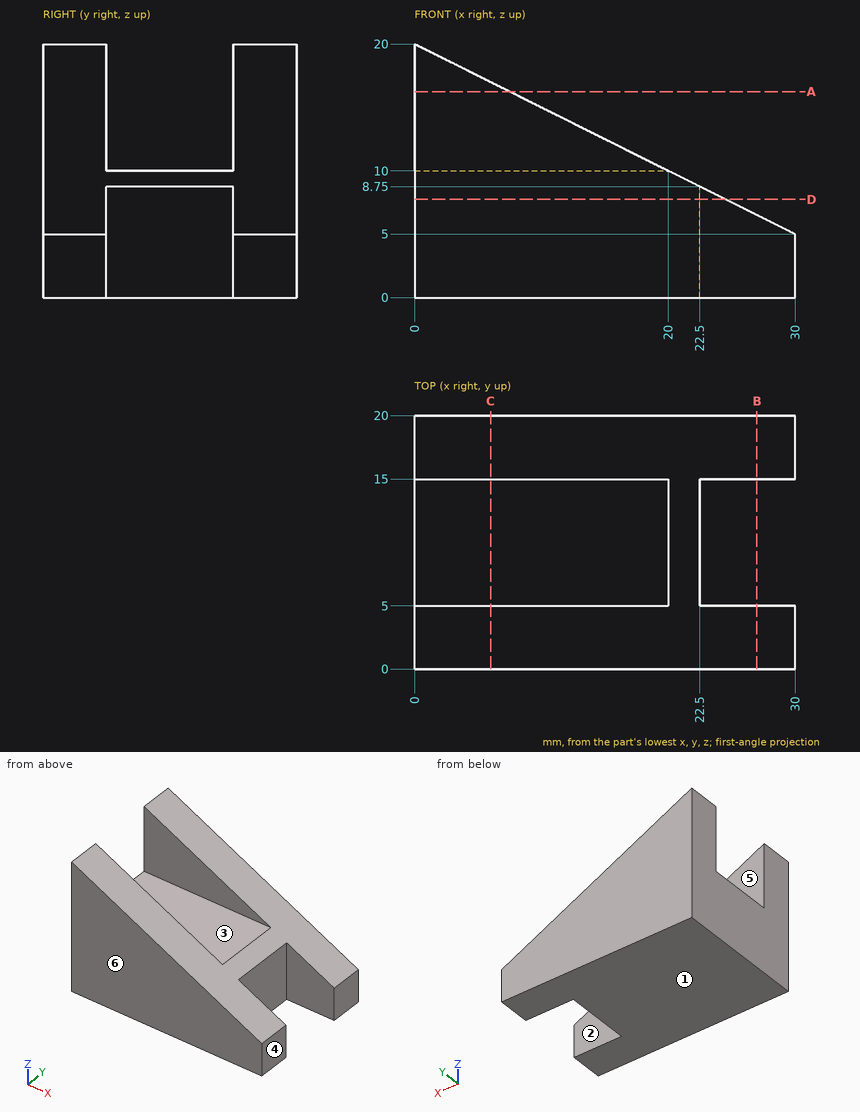
Answer from the drawing. Dimensions are ordinates in mm from the lowest x, y and z of the part. A direction names the side the tool comes from. Round coordinates to 2 decimals unless told otherwise and drop trailing zeros. Write each loop counter-clockwise with the first axis right and the second up, starting at its lowest first coordinate (ties: lowest second). Pieces come first, ordered by that corner, then holes.
1. Given pin 1 Ø8 at (x, y) = (11.5, 11.5) entering from +Z; pin 2 Ø3 at (x, y) = (26, 3.5) entering from +Z; pin 3 Ø2 at (x, y) = (19.5, 10) entering from +Z, each flat-ended and moving along its own axis, determine where each tip first touches the part or whether it passes through.
2. The part is cut by section B-B, the plane x = 27. Determine the outline of the cut face in (y, z), then the cut area to 3 significant figures.
3. Straight lines are drawn through the part: L1, parallel to Y at x = 10, z = 14.5; L2, parallel to Z at x = 18, y = 14; L3, parallel to X at y = 8.75, z = 4.5. For each, find the intervals that lie inside material, in ascending order.
4. The part is cut by section D-D, the plane z = 7.75. Determine the outline of the cut face in (x, y), then the cut area to 3 significant figures.
5. The part is cut by section C-C, the plane x = 6. Determine the outline of the cut face in (y, z).
6. The part is cut by section A-A, the plane z = 16.25. Determine the outline of the cut face in (x, y), then the cut area to 3 significant figures.
7. Which of the six approach directions +Z, -Z, +X, -X, +Y, -Y give full straight-line access (tool end or side, diameter ignored) to the marked faces 1, 2 and 3?
8. Determine the mould class of the marked faces 4, 5 and 6 for opening direction Y: pulls with the +Y half, pulls with the -Y half, needs draft (parallel to the pull), parting line crosses it, or undercut.
Values:
1. pin 1: stops at z = 15.22
1. pin 2: stops at z = 7.75
1. pin 3: stops at z = 10
2. outline: (0, 0) - (5, 0) - (5, 6.5) - (0, 6.5) - close; (15, 0) - (20, 0) - (20, 6.5) - (15, 6.5) - close
2. area: 65.0 mm2
3. L1: y = 0 to 5, 15 to 20
3. L2: z = 0 to 10
3. L3: x = 0 to 22.5
4. outline: (0, 0) - (24.5, 0) - (24.5, 5) - (22.5, 5) - (22.5, 15) - (24.5, 15) - (24.5, 20) - (0, 20) - close
4. area: 470 mm2
5. outline: (0, 0) - (20, 0) - (20, 17) - (15, 17) - (15, 10) - (5, 10) - (5, 17) - (0, 17) - close
6. outline: (0, 0) - (7.5, 0) - (7.5, 5) - (0, 5) - close; (0, 15) - (7.5, 15) - (7.5, 20) - (0, 20) - close
6. area: 75.0 mm2
7. face 1: -Z, +X, -X, +Y, -Y
7. face 2: +Z, -Z, +X
7. face 3: +Z, +X, -X
8. face 4: needs draft
8. face 5: undercut
8. face 6: pulls with the -Y half
